Can you work these out from the model? Positions are in its coordinate system, mm. Give positions to 0.01 mm unless a question says otherwise; leave off trailing zeros. Order: outer loops, then holes, each group sorted by start corner. A loop starts at its lowest first (then second) coordinate and runs counter-clockwise, first axis right, second up. Notation, with made-up numbers: (-15, 52.5) - (-9, 52.5) arc R15 ccw to (-9, 61.5) - close; hole circle Ø7 at (76.5, -10). An arc over 180 degrees is marked (long way). Return JSON: item names as keys, results as strings.
Autodesk Inventor part; units mm, degrees
ref_plane "YZ Plane" through (0, 0, 0) normal (1, 0, 0) x (0, 1, 0)
ref_plane "XZ Plane" through (0, 0, 0) normal (0, 1, 0) x (-1, 0, 0)
ref_plane "XY Plane" through (0, 0, 0) normal (0, 0, 1) x (1, 0, 0)
sketch "Sketch1" plane through (0, 0, 0) normal (0, 0, 1) x (1, 0, 0)
  circle A0 centre (0, 0) radius 5
  circle A1 centre (0, 0) radius 25
  line L0 (25, 0) -> (-25, 0)
  line L1 (-25, 0) -> (-25, 200)
  line L2 (-25, 200) -> (25, 200)
  line L3 (25, 200) -> (25, 0)
  dimension "d1" = 50
  dimension "d0" = 10
  dimension "d2" = 200
extrude "Extrusion1" add sketch "Sketch1" along normal blind 50 contours L0 A1 A0 | A0 L0 A1 | A1 L1 L2 L3
sketch "Sketch2" plane through (-25, 200, 0) normal (0, 1, 0) x (1, 0, 0)
  line L0 (50, 0) -> (0, 0)
  line L1 (0, 0) -> (0, -50)
  point P0 (25, 0)
  point P1 (25, -25)
  dimension "d5" = 25
  dimension "d6" = 25
hole "Hole1" at (0, 200, 25) direction (0, -1, 0) diameter 10 depth 8 tip angle 118
properties part number "link5"
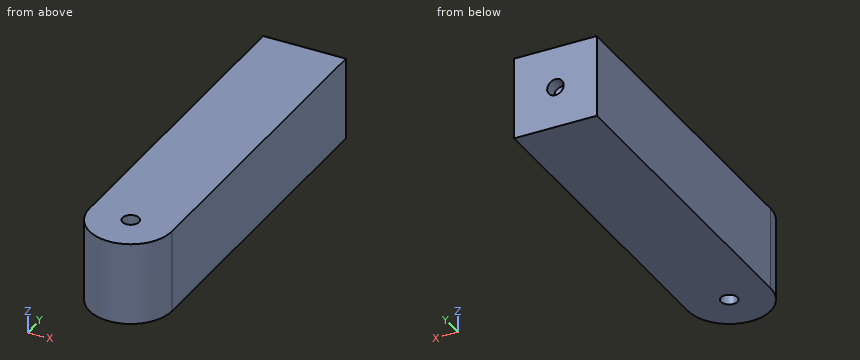
1. For pin 1 Ø6 at (x, z) = (2, 16.5) entering from -Y; pin 2 Ø4 at (x, z) = (-17.5, 5.5) entering from -Y; pin 3 Ø8 at (x, y) = (0, 0) entering from -Z; pin 4 Ø4 at (x, z) = (4.5, 19.5) entering from -Y, each with a flat end and sliding along its axis, tell me the tip position at first contact or that it passes through.
Checks:
{"pin 1": "y = -25", "pin 2": "y = -19.62", "pin 3": "through", "pin 4": "y = -24.87"}
2. Suppose I cut it at B-B (x = -21.5). List the corners of the cut face in (y, z) for me, plus the area to 3 significant figures.
Checks:
{"outline": "(-12.76, 0) - (200, 0) - (200, 50) - (-12.76, 50) - close", "area": "10,600 mm^2"}
3. Suppose I cut it at A-A (z = 33). List the corners of the cut face in (x, y) for me, plus the area to 3 significant figures.
Checks:
{"outline": "(-25, 0) arc R25 ccw to (25, 0) - (25, 200) - (-25, 200) - close; hole circle Ø10 at (0, 0)", "area": "10,900 mm^2"}
4. If I drill on L1, parallel to X at y = 0, z = 33; L2, parallel to Z at x = 0, y = 195.25; L3, parallel to X at y = 2, z = 37, over which ranges is the centre line in solid material (lowest first)? Write a range as [from, to].
Checks:
{"L1": "[-25, -5], [5, 25]", "L2": "[0, 20], [30, 50]", "L3": "[-25, -4.58], [4.58, 25]"}
